Read the model definition and answer for the solid it produces. Units are mm, in the model's axes. Face numbers are marked on the shaded views. A direction names the side the tool comes from. Coordinates: 2 decimals unless noted, no trailing zeros. Write each loop counter-clockwise with the first axis right and the second up, starting at its lowest first coordinate (ties: lowest second). Pieces come first, ordered by that corner, then holes.
Item 1: Section C-C (y = -21) is taken. Give the vertices of the cut face in (x, z), then the cut area to 3 significant figures.
Item 2: Section A-A (x = 0) is taken. Give the vertices of the cut face in (y, z).
Item 3: Each of these flat-tipped pins is pushed along its axis until it touches: P1, Ø10, axis at x = -70, z = 10.5, coming from the -Y side; P2, Ø12, axis at x = 2.5, y = -24, coming from the +Z side; P3, Ø5, axis at x = 6.5, y = -28, coming from the +Z side. Where does it stop, or does it pass through?
Item 4: Section D-D (x = 59) is taken. Give the vertices of the cut face in (y, z), then the cut area to 3 significant figures.
Item 5: Straight lines are drawn through the part: probe 1 along Z at (x, y) = (0, -26); probe 2 along Y at (x, z) = (-77.5, 43.5); probe 3 along X at (y, z) = (-2, 18.5). For each, find the intervals that lie inside material, in ascending order.
Item 6: Section B-B (z = 0) is taken. Give the vertices of the cut face in (x, y), then the cut area to 3 significant figures.
Item 7: Determine the mould class of the marked faces 1, 2 and 3 for opening direction X: released by +X, released by -X, zero draft, split by the parting line, or undercut.
Item 8: A tool of negligible diameter and unlimited length cuts with its end or side. For the marked faces 4 and 5, from which of +Z, -Z, +X, -X, +Y, -Y can it reach the whole face along a straight path? Write none if from no direction.
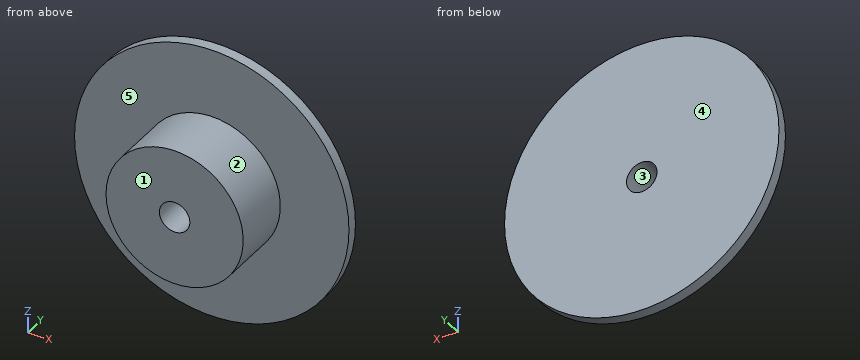
Autodesk Inventor part; units mm, degrees
ref_plane "YZ Plane" through (0, 0, 0) normal (1, 0, 0) x (0, 1, 0)
ref_plane "XZ Plane" through (0, 0, 0) normal (0, 1, 0) x (-1, 0, 0)
ref_plane "XY Plane" through (0, 0, 0) normal (0, 0, 1) x (1, 0, 0)
sketch "Sketch1" plane through (0, 0, 0) normal (0, 1, 0) x (-1, 0, 0)
  circle A0 centre (0, 0) radius 90
  circle A1 centre (0, 0) radius 45
  circle A2 centre (0, 0) radius 10
  dimension "d0" = 180
  dimension "d1" = 90
  dimension "d2" = 20
extrude "Extrusion1" add sketch "Sketch1" along normal blind 7 contours A0 | A1
extrude "Extrusion2" add sketch "Sketch1" against normal blind 40 contours A1
properties part number "56T-Sprocket"
Established:
1. outline: circle Ø90 at (0, 0); hole circle Ø20 at (0, 0)
1. area: 6,050 mm2
2. outline: (-40, -45) - (0, -45) - (0, -90) - (7, -90) - (7, -10) - (-40, -10) - close; (-40, 10) - (7, 10) - (7, 90) - (0, 90) - (0, 45) - (-40, 45) - close
3. P1: stops at y = 0
3. P2: stops at z = 45
3. P3: stops at z = 44.82
4. outline: (0, -67.96) - (7, -67.96) - (7, 67.96) - (0, 67.96) - close
4. area: 951 mm2
5. probe 1: z = -45 to -10, 10 to 45
5. probe 2: y = 0 to 7
5. probe 3: x = -41.02 to 41.02
6. outline: (-90, 0) - (-45, 0) - (-45, -40) - (-10, -40) - (-10, 7) - (-90, 7) - close; (10, -40) - (45, -40) - (45, 0) - (90, 0) - (90, 7) - (10, 7) - close
6. area: 3,920 mm2
7. face 1: zero draft
7. face 2: split by the parting line
7. face 3: undercut
8. face 4: +Z, -Z, +X, -X, +Y
8. face 5: -Y
